Design review of the part built by this model. Coordinates are the model's own, in mm. Face numbers are marked on the shaded views. Give positions to 0.01 mm unless a question says otherwise; leave off trailing zeros. Loops run counter-clockwise (first coordinate to the right, second up) from the corner with the lowest first, then second, coordinate; pieces in that order, holes last. Notation, with made-up numbers: (60.25, 66) -> (97.25, 66) arc R16 cw to (97.25, 97) -> close; hole circle Ø7 at (-37, 31.25). An arc over 180 degrees is marked (long way). Use CSV: the item, a comma, the result in double quotes. Start each with the question number.
Item 1: We need section D-D (z = 60). State the section outline as (x, y) points, plus the area to 3 significant figures.
Item 2: We need section C-C (y = -9). State the section outline as (x, z) points.
Item 3: We need section B-B (z = 6). State the section outline as (x, y) points.
Item 4: The part is to be moulded in two halves that separate along X. For the marked faces 1, 2 and 3, say which applies: +X half, -X half, draft (parallel to the pull), parting line (faces both ways), or undercut.
Item 5: Clearance check with flat-ended pins moving along their axes: pin 1 (6 mm diameter, centred on x = 1.5, z = 63.5, fed in from -Y); pin 2 (5 mm diameter, centred on x = 3, z = 64, fed in from +Y). State where each tip first meets the part, or that it passes through.
Item 6: We need section A-A (x = 0). State the section outline as (y, z) points.
Item 7: Wall thickness on line 1 along Z through (x, y) = (0, -4.5); line 2 along X through (y, z) = (-10, 11.5); line 3 along X through (y, z) = (-9.5, 11): over which ranges is each line inside the solid? List them lowest first. Write a range as from..to.
from build123d import *

# Parameters (mm, degrees)
F0_R     = 6.35
F1_DEPTH = 12.7
F2_SIZE  = 1.5


with BuildPart() as f1:
    # F0 (on Front) → F1 (new body)
    with BuildSketch(Plane.XZ):
        with BuildLine():
            Line((20, 0), (9.36164, 75.695866))
            ThreePointArc((9.36164, 75.695866), (7.690595, 78.773548), (4.4103, 80))
            Line((4.4103, 80), (-4.4103, 80))
            ThreePointArc((-4.4103, 80), (-7.690595, 78.773548), (-9.36164, 75.695866))
            Line((-9.36164, 75.695866), (-20, 0))
            Line((-20, 0), (-15, 0))
            ThreePointArc((-15, 0), (0, 15), (15, 0))
            Line((15, 0), (20, 0))
        make_face()
        with Locations((0, 60)):
            Circle(F0_R, mode=Mode.SUBTRACT)
    extrude(amount=F1_DEPTH)

    # F2
    f2_edges = [f1.edges().sort_by_distance(p)[0] for p in [
        (-6.35, -12.7, 60),
        (-6.35, 0, 60),
    ]]
    chamfer(f2_edges, length=F2_SIZE)


solid = f1.part
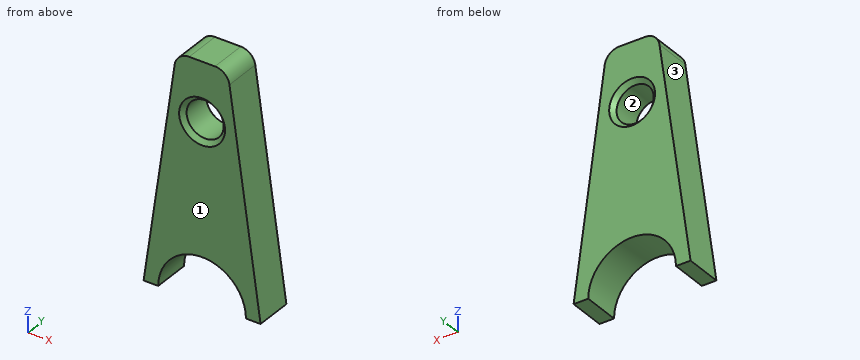
Results found:
1,outline,"(-11.57, -12.7) -> (-7.85, -12.7) -> (-6.35, -11.2) -> (-6.35, -1.5) -> (-7.85, 0) -> (-11.57, 0) -> close; (6.35, -11.2) -> (7.85, -12.7) -> (11.57, -12.7) -> (11.57, 0) -> (7.85, 0) -> (6.35, -1.5) -> close"
1,area,"128 mm²"
2,outline,"(-20, 0) -> (-15, 0) arc R15 cw to (15, 0) -> (20, 0) -> (9.36, 75.7) arc R5 ccw to (4.41, 80) -> (-4.41, 80) arc R5 ccw to (-9.36, 75.7) -> close; hole circle Ø12.7 at (0, 60)"
3,outline,"(-19.16, -12.7) -> (-13.75, -12.7) -> (-13.75, 0) -> (-19.16, 0) -> close; (13.75, -12.7) -> (19.16, -12.7) -> (19.16, 0) -> (13.75, 0) -> close"
4,face 1,"draft"
4,face 2,"undercut"
4,face 3,"-X half"
5,pin 1,"y = -11.66"
5,pin 2,"y = -0.35"
6,outline,"(-12.7, 15) -> (0, 15) -> (0, 52.15) -> (-1.5, 53.65) -> (-11.2, 53.65) -> (-12.7, 52.15) -> close; (-12.7, 67.85) -> (-11.2, 66.35) -> (-1.5, 66.35) -> (0, 67.85) -> (0, 80) -> (-12.7, 80) -> close"
7,line 1,"15..53.65, 66.35..80"
7,line 2,"-18.38..-9.63, 9.63..18.38"
7,line 3,"-18.45..-10.2, 10.2..18.45"
